The listing builds one solid part. Answer for the finished solid, in the listing's coordinates (mm). A direction names the side the tool comes from. Round coordinates to 2 decimals unless told otherwise and drop trailing zeros. Order: outer loops, then holes, each group sorted by start corner. A loop starts at its lowest first (then second) coordinate and runs counter-clockwise, first axis right, second up. Notation, with made-up numbers: (-33.5, -33) - (-2.5, -33) arc R25 ccw to (-2.5, 0) - close; hole circle Ø10 at (23, 78.25). An arc over 180 degrees is marked (long way). One line per item, written item: value. Start each with the question number.
1. For a pull along Z with two mould halves and no side action, classify faces 1 (the cylindrical face through (0.99, 8.25, 0.03)), 2 (the cylindrical face through (0.986, 0.192, 15.212)), 3 (the flat face through (0.99, -2.28, -8.31)), 4 (the cylindrical face through (0.986, -6.262, -0.108)) as released by +Z, released by -Z, zero draft, split by the parting line, or undercut.
2. Section A-A, the plane y = 4.75 is taken. Give the vertices of the cut face in (x, z).
3. Section C-C, the plane z = 0 is taken. Count the separate pieces of the cut face and the enclosed holes in it, then the cut area to 3 significant figures.
4. Straight lines are drawn through the part: line 1 (Y direction, x = -1.35, z = 0); line 2 (X direction, y = 0.75, z = 6.5); line 3 (Y direction, x = 0.05, z = 4.5). For each, find the intervals that lie inside material, in ascending order.
5. Section D-D, the plane x = -1.5 is taken. Give the vertices of the cut face in (y, z), then the cut area to 3 significant figures.
6. Section B-B, the plane z = -12.75 is taken. Give the vertices of the cut face in (x, y), then the cut area to 3 significant figures.
7. Flat-ended cylindrical pins translate along their axes: P1, Ø2, axis at x = 1.5, z = 5.5, coming from the -Y side; P2, Ø4, axis at y = 0, z = 0, coming from the +X side; P3, Ø1, axis at x = 1, y = -4.5, coming from the -Z side; P4, Ø3, axis at y = 5, z = 7, coming from the +X side. Find the tip coordinate at first contact, or state that the pin passes through.
8. A tool of negligible diameter and unlimited length cuts with its end or side. For faces 5 (the cylindrical face through (1.76, -1.52, -1.66)), 6 (the cylindrical face through (0.986, 0.192, 9.212)), 7 (the flat face through (1, 5, -1.5)), from which of +Z, -Z, +X, -X, +Y, -Y can it reach the whole face along a straight path? Write none if from no direction.
from build123d import *

# Parameters (mm, degrees)
SKETCH_1_R          = 3.25
SKETCH_1_R_2        = 0.5
EXTRUDE_1_DEPTH     = 2
EXTRUDE_START       = -2
SKETCH_2_R          = 3.25
SKETCH_2_R_2        = 1.25
EXTRUDE_2_DEPTH     = 2
SKETCH_3_R          = 3.25
SKETCH_3_R_2        = 2.25
EXTRUDE_3_DEPTH     = 2
EXTRUDE_START_2     = 0.5
SKETCH_4_R          = 3.25
SKETCH_4_R_2        = 2.25
EXTRUDE_5_DEPTH     = 0.5
SKETCH_5_R          = 2.25
SKETCH_5_R_2        = 1.25
CUT_EXTRUDE_1_DEPTH = 1


with BuildPart() as part:
    # 草图1 → 凸台-拉伸1 (new body)
    with BuildSketch(Plane(origin=(0, 0, 0), x_dir=(0, 0, -1), z_dir=(1, 0, 0))):
        with BuildLine():
            Line((-14.927966102, 1.489405273), (-1.5, 3.093886487))
            Line((-1.5, 3.093886487), (-1.5, 6.75))
            ThreePointArc((-1.5, 6.75), (0, 8.25), (1.5, 6.75))
            Line((1.5, 6.75), (1.5, 3.093886487))
            Line((1.5, 3.093886487), (14.927966102, 1.489405273))
            ThreePointArc((14.927966102, 1.489405273), (16.25, 0), (14.927966102, -1.489405273))
            Line((14.927966102, -1.489405273), (1.5, -3.093886487))
            Line((1.5, -3.093886487), (1.5, -6.75))
            ThreePointArc((1.5, -6.75), (0, -8.25), (-1.5, -6.75))
            Line((-1.5, -6.75), (-1.5, -3.093886487))
            Line((-1.5, -3.093886487), (-14.927966102, -1.489405273))
            ThreePointArc((-14.927966102, -1.489405273), (-16.25, 0), (-14.927966102, 1.489405273))
        make_face()
        Circle(SKETCH_1_R, mode=Mode.SUBTRACT)
        with Locations((4.75, 0)):
            Circle(SKETCH_1_R_2, mode=Mode.SUBTRACT)
        with Locations((6.75, 0)):
            Circle(SKETCH_1_R_2, mode=Mode.SUBTRACT)
        with Locations((8.75, 0)):
            Circle(SKETCH_1_R_2, mode=Mode.SUBTRACT)
        with Locations((10.75, 0)):
            Circle(SKETCH_1_R_2, mode=Mode.SUBTRACT)
        with Locations((12.75, 0)):
            Circle(SKETCH_1_R_2, mode=Mode.SUBTRACT)
        with Locations((14.75, 0)):
            Circle(SKETCH_1_R_2, mode=Mode.SUBTRACT)
        with Locations(Location((-14.75, 0, 0), (0, 0, 180))):
            Circle(SKETCH_1_R_2, mode=Mode.SUBTRACT)
        with Locations(Location((-12.75, 0, 0), (0, 0, 180))):
            Circle(SKETCH_1_R_2, mode=Mode.SUBTRACT)
        with Locations(Location((-10.75, 0, 0), (0, 0, 180))):
            Circle(SKETCH_1_R_2, mode=Mode.SUBTRACT)
        with Locations(Location((-8.75, 0, 0), (0, 0, 180))):
            Circle(SKETCH_1_R_2, mode=Mode.SUBTRACT)
        with Locations(Location((-6.75, 0, 0), (0, 0, 180))):
            Circle(SKETCH_1_R_2, mode=Mode.SUBTRACT)
        with Locations(Location((-4.75, 0, 0), (0, 0, 180))):
            Circle(SKETCH_1_R_2, mode=Mode.SUBTRACT)
        with Locations((0, 4.75)):
            Circle(SKETCH_1_R_2, mode=Mode.SUBTRACT)
        with Locations((0, 6.75)):
            Circle(SKETCH_1_R_2, mode=Mode.SUBTRACT)
        with Locations(Location((0, -4.75, 0), (0, 0, 180))):
            Circle(SKETCH_1_R_2, mode=Mode.SUBTRACT)
        with Locations(Location((0, -6.75, 0), (0, 0, 180))):
            Circle(SKETCH_1_R_2, mode=Mode.SUBTRACT)
    extrude(amount=EXTRUDE_1_DEPTH)

    # 草图2 → 凸台-拉伸2 (add)
    with BuildSketch(Plane(origin=(2, 0, 0), x_dir=(0, 0, -1), z_dir=(1, 0, 0)).offset(EXTRUDE_START)):
        Circle(SKETCH_2_R)
        Circle(SKETCH_2_R_2, mode=Mode.SUBTRACT)
    extrude(amount=EXTRUDE_2_DEPTH)

    # 草图3 → 凸台-拉伸3 (add)
    with BuildSketch(Plane.ZY):
        with Locations(Location((0, 0, 0), (0, 0, 180))):
            Circle(SKETCH_3_R)
        Circle(SKETCH_3_R_2, mode=Mode.SUBTRACT)
    extrude(amount=EXTRUDE_3_DEPTH)

    # 草图4 → 凸台-拉伸5 (add)
    with BuildSketch(Plane(origin=(2, 0, 0), x_dir=(0, 0, -1), z_dir=(1, 0, 0)).offset(EXTRUDE_START_2)):
        Circle(SKETCH_4_R)
        with Locations(Location((0, 0, 0), (0, 0, 180))):
            Circle(SKETCH_4_R_2, mode=Mode.SUBTRACT)
    extrude(amount=-EXTRUDE_5_DEPTH)

    # 草图5 → 切除-拉伸1 (cut)
    with BuildSketch(Plane(origin=(2, 0, 0), x_dir=(0, 0, -1), z_dir=(1, 0, 0))):
        with Locations(Location((0, 0, 0), (0, 0, 180))):
            Circle(SKETCH_5_R)
        Circle(SKETCH_5_R_2, mode=Mode.SUBTRACT)
    extrude(amount=-CUT_EXTRUDE_1_DEPTH, mode=Mode.SUBTRACT)


solid = part.part
Answer list:
1. face 1: split by the parting line
1. face 2: undercut
1. face 3: released by -Z
1. face 4: undercut
2. outline: (0, -1.5) - (2, -1.5) - (2, -0.5) - (0, -0.5) - close; (0, 0.5) - (2, 0.5) - (2, 1.5) - (0, 1.5) - close
3. separate pieces: 6
3. enclosed holes: 0
3. area: 23.0 mm²
4. line 1: y = -3.25 to -2.25, 2.25 to 3.25
4. line 2: x = 0 to 2
4. line 3: y = -2.74 to -0.43, 0.43 to 2.74
5. outline: circle Ø6.5 at (0, 0); hole circle Ø4.5 at (0, 0)
5. area: 17.3 mm²
6. outline: (0, -1.75) - (2, -1.75) - (2, -0.5) - (0, -0.5) - close; (0, 0.5) - (2, 0.5) - (2, 1.75) - (0, 1.75) - close
6. area: 5.00 mm²
7. P1: stops at y = -2.74
7. P2: stops at x = 1
7. P3: stops at z = -1.5
7. P4: passes through
8. face 5: +X
8. face 6: +X, -X
8. face 7: -Z, +X, -X, +Y
